```python
from build123d import *

# Parameters (mm, degrees)
SKIZZE1_R                       = 16
AUFSATZ_LINEAR_AUSTRAGEN1_DEPTH = 2.725
DURCHGANGSLOCH_F_R_M41_D        = 4.5
FASE1_SIZE                      = 0.5


with BuildPart() as part:
    # Skizze1 → Aufsatz-Linear austragen1 (new, symmetric)
    with BuildSketch(Plane.XY):
        Circle(SKIZZE1_R)
    extrude(amount=AUFSATZ_LINEAR_AUSTRAGEN1_DEPTH, both=True)

    # Durchgangsloch für M41 (through all)
    with Locations(Plane.XY.offset(2.725)):
        with Locations((-10.392304845, 6), (0, 12), (10.392304845, 6), (10.392304845, -6), (0, -12), (-10.392304845, -6)):
            Hole(DURCHGANGSLOCH_F_R_M41_D / 2)

    # Fase1
    fase1_edges = [part.edges().sort_by_distance(p)[0] for p in [
        (-16, 0, -2.725),
        (-16, 0, 2.725),
    ]]
    chamfer(fase1_edges, length=FASE1_SIZE)


solid = part.part
```
The model under review builds one solid part; all positions refer to its coordinate system, in mm. Round coordinates to 2 decimals unless told otherwise and drop trailing zeros. Write each loop counter-clockwise with the first axis right and the second up, starting at its lowest first coordinate (ties: lowest second). Pieces come first, ordered by that corner, then holes. Notation, with made-up numbers: M 84.25,64 L 116.25,64 A27 ccw 116.25,94 Z; hole C 7.25,32 d8. An arc over 180 degrees is marked long. Use CSV: the item, a comma, the result in double quotes. Start each with the question number.
(1) We need section A-A, the plane x = 0. State the section outline as (y, z) points (3 decimals), then the cut area to 3 significant figures.
(2) Clearance check with flat-ended pins moving along their axes: P1, Ø3, axis at x = 3.5, z = 1, coming from the -Y side; P2, Ø1.5, axis at x = 5, z = 2, coming from the +Y side; P3, Ø1, axis at y = -8, z = 2, coming from the +X side; P4, Ø2.5, axis at x = 0, y = -12, coming from the +Z side. State where each tip first meets the part, or that it passes through.
(3) For line 1 along Y through (x, z) = (0, 0.25); line 2 along Y through (x, z) = (9.5, -0.15); line 3 along X through (y, z) = (-4.5, -2.2), list the stretches that pass through material, from the lowest coordinate up.
(4) The part is to be moulded in two halves that separate along X. For faces 1 (the face through (-3.47, -15.62, 0.03)), 2 (the face through (-8.144, -5.901, -0.038)), 3 (the face through (0, 0, 2.725)), say which applies: +X half, -X half, draft (parallel to the pull), parting line (faces both ways), or undercut.
(5) We need section B-B, the plane z = -1.3. State the section outline as (x, y) points.
(6) We need section C-C, the plane y = 6. State how many separate pieces and enclosed holes the cut face has, then the cut area to 3 significant figures.
Findings:
1,outline,"M -16,-2.225 L -15.5,-2.725 L -14.25,-2.725 L -14.25,2.725 L -15.5,2.725 L -16,2.225 Z; M -9.75,-2.725 L 9.75,-2.725 L 9.75,2.725 L -9.75,2.725 Z; M 14.25,-2.725 L 15.5,-2.725 L 16,-2.225 L 16,2.225 L 15.5,2.725 L 14.25,2.725 Z"
1,area,"125 mm^2"
2,P1,"y = -15.87"
2,P2,"y = 15.43"
2,P3,"x = 14.13"
2,P4,"through"
3,line 1,"-16 to -14.25, -9.75 to 9.75, 14.25 to 16"
3,line 2,"-12.87 to -8.07, -3.93 to 3.93, 8.07 to 12.87"
3,line 3,"-15.35 to -12.07, -8.72 to 8.72, 12.07 to 15.35"
4,face 1,"parting line"
4,face 2,"undercut"
4,face 3,"draft"
5,outline,"C 0,0 d32; hole C -10.39,-6 d4.5; hole C -10.39,6 d4.5; hole C 0,-12 d4.5; hole C 0,12 d4.5; hole C 10.39,-6 d4.5; hole C 10.39,6 d4.5"
6,separate pieces,"3"
6,enclosed holes,"0"
6,area,"112 mm^2"
